Input: part model. Units: mm. Frame: model coordinates. A direction names the side the tool comes from. Give positions to 0.01 mm unless a question says otherwise; leave off trailing zeros. Write each loop counter-clockwise with the first axis right and the second up, starting at its lowest first coordinate (ties: lowest second). Pieces come first, ordered by that corner, then holes.
Solid Edge part; units mm, degrees
sketch "Sketch1" plane through (0, 0, 0) normal (0, 0, 1) x (1, 0, 0)
  line L0 (-10, 45) -> (-10, 27)
  line L1 (10, 27) -> (10, 45)
  line L2 (30, 45) -> (10, 45)
  line L3 (30, -45) -> (30, 45)
  line L4 (-30, -45) -> (30, -45)
  line L5 (-30, 45) -> (-30, -45)
  line L6 (-10, 45) -> (-30, 45)
  arc A0 (10, 27) -> (-10, 27) centre (0, 27) cw
extrude "Protrusion1" add sketch "Sketch1" along normal blind 20
sketch "Sketch2" plane through (0, -45, 10) normal (0, -1, 0) x (1, 0, 0)
  line L0 (30, 35) -> (30, 10)
  line L1 (10, 35) -> (30, 35)
  line L2 (-30, 35) -> (-10, 35)
  line L3 (-30, 10) -> (-30, 35)
  arc A0 (-10, 35) -> (10, 35) centre (0, 35) cw
extrude "ExtrudedProtrusion_2" add sketch "Sketch2" against normal blind 35 material side at (30.05, -45, 32.5)
Q1. Section D-D, the plane y = -2. Return the cut outline in (x, z).
Q2. Section B-B, the plane x = -24.5. Return the cut outline in (y, z).
Q3. Section C-C, the plane z = 10. Return the cut outline in (x, y), then the cut area to 3 significant figures.
Q4. Access query for faces 1 (the flat face through (-20, -28, 45)), 2 (the flat face through (-10, 36, 10)), 3 (the flat face through (0, -45, 21)), 4 (the flat face through (0, -10, 33)), 5 (the flat face through (20, -28, 45)). Directions: +Z, -Z, +X, -X, +Y, -Y. A direction counts if a zero-diameter tool reaches every point of the face in a straight line with its end or side. Return the directions, or none.
Q5. Section A-A, the plane y = 19. Return the cut outline in (x, z), then the cut area to 3 significant figures.
Q6. Material intervals for line 1 along X through (y, z) = (29, 10.5); line 2 along Z through (x, y) = (-23.5, -23); line 3 along X through (y, z) = (22.5, 12.5), sorted ascending.
Q7. Mould query, pull axis X, two halves, no side actions, for faces 6 (the flat face through (-20, 45, 10)), 7 (the cylindrical face through (0, -28, 55)), 8 (the flat face through (10, 36, 10)). Classes: +X half, -X half, draft (parallel to the pull), parting line (faces both ways), or undercut.
Q8. Pin query (flat end, axial travel): pin 1 (10 mm diameter, centred on x = 17, y = -26.5, fed in from +Z); pin 2 (12 mm diameter, centred on x = -8.5, y = 22.5, fed in from +Z); pin 3 (17.5 mm diameter, centred on x = 5, z = 31.5, fed in from +Y). Return the tip coordinate at first contact, or that it passes through.
Solutions:
1. outline: (-30, 0) - (30, 0) - (30, 20) - (-30, 20) - close
2. outline: (-45, 0) - (45, 0) - (45, 20) - (-10, 20) - (-10, 45) - (-45, 45) - close
3. outline: (-30, -45) - (30, -45) - (30, 45) - (10, 45) - (10, 27) arc R10 cw to (-10, 27) - (-10, 45) - (-30, 45) - close
3. area: 4,880 mm2
4. face 1: +Z, -X, +Y, -Y
4. face 2: +Z, -Z, +Y
4. face 3: +Z, -Z, +X, -X, -Y
4. face 4: +Z, +X, -X, +Y
4. face 5: +Z, +X, +Y, -Y
5. outline: (-30, 0) - (-6, 0) - (-6, 20) - (-30, 20) - close; (6, 0) - (30, 0) - (30, 20) - (6, 20) - close
5. area: 960 mm2
6. line 1: x = -30 to -10, 10 to 30
6. line 2: z = 0 to 45
6. line 3: x = -30 to -8.93, 8.93 to 30
7. face 6: draft
7. face 7: parting line
7. face 8: undercut
8. pin 1: stops at z = 45
8. pin 2: stops at z = 20
8. pin 3: stops at y = -10
